Verification items for the finished model (mm, model axes). A direction names the side the tool comes from. Round coordinates to 2 decimals unless told otherwise and drop trailing zeros. Write each loop counter-clockwise with the first axis right and the second up, starting at its lowest first coordinate (ties: lowest second). Pieces come first, ordered by that corner, then holes. Notation, with made-up numbers: M 32,17.25 L 58,17.25 A36 cw 58,52.25 Z; hole C -23,26 d3. An arc over 180 degrees is marked long. One line per question, with ' | ' between items. Start each with the question number.
Q1. Thickness scan on line 1 along Z through (x, y) = (7, -0.3); line 2 along X through (y, z) = (0.5, 9.25); line 3 along X through (y, z) = (11, 3). Record the ranges inside material, lowest first. Write a range as from..to.
Q2. Cross-section at D-D (y = 8). Record the boundary of the cut face in (x, z), then the cut area to 3 significant figures.
Q3. Cross-section at A-A (z = 7.5). State how many separate pieces and enclosed holes the cut face has, then the cut area to 3 significant figures.
Q4. Cross-section at B-B (x = -7.75). Record the boundary of the cut face in (y, z), then the cut area to 3 significant figures.
Q5. Cross-section at C-C (z = 1). Record the boundary of the cut face in (x, y).
Q6. Gauge pin test, flat ends, axial feed: pin 1 (8 mm diameter, centred on x = -7.5, z = 9, fed in from -Y); pin 2 (3.5 mm diameter, centred on y = 9, z = 6, fed in from -X); pin 3 (3 mm diameter, centred on y = 18, z = 2, fed in from -X); pin 4 (3 mm diameter, centred on y = 19.5, z = 7.5, fed in from -X). Record the tip position at first contact, or that the pin passes through.
Q7. Release check for a two-part mould opening along X. For faces 5 (the face through (-0.1, 18.4, 7.4)), 6 (the face through (11, 0, 7)), 7 (the face through (7, 23.5, 7)) record: released by +X, released by -X, zero draft, split by the parting line, or undercut.
Q8. Tool access check on faces 1 (the face through (-3.5, 9, 7)), 2 (the face through (-11, 0, 7)), 3 (the face through (8.18, -0.03, 5.24)), 4 (the face through (9.4, 2, 5.7)). Record the directions out of +Z, -Z, +X, -X, +Y, -Y that give a thin tool (end or side, any length) a straight path to the whole face; none if there is none.
from build123d import *

# Parameters (mm, degrees)
SALIENTE_EXTRUIR1_DEPTH = 15
REDONDEO1_R             = 0.5
REDONDEO2_R             = 0.5
CROQUIS3_R              = 2.55
CORTAR_EXTRUIR1_DEPTH   = 6


with BuildPart() as part:
    # Croquis1 → Saliente-Extruir1 (new body)
    with BuildSketch(Plane.XY):
        with BuildLine():
            Line((-11, 2), (-3.5, 2))
            Line((-3.5, 2), (-3.5, 15.1))
            ThreePointArc((-3.5, 15.1), (-7.571657678, 18.452228214), (-9.1, 23.5))
            Line((-9.1, 23.5), (-5.1, 23.5))
            ThreePointArc((-5.1, 23.5), (0, 18.4), (5.1, 23.5))
            Line((5.1, 23.5), (9.1, 23.5))
            ThreePointArc((9.1, 23.5), (7.571657678, 18.452228214), (3.5, 15.1))
            Line((3.5, 15.1), (3.5, 2))
            Line((3.5, 2), (11, 2))
            Line((11, 2), (11, -2))
            Line((11, -2), (-11, -2))
            Line((-11, -2), (-11, 2))
        make_face()
    extrude(amount=SALIENTE_EXTRUIR1_DEPTH)

    # Redondeo1
    redondeo1_edges = [part.edges().sort_by_distance(p)[0] for p in [
        (-3.5, 2, 7.5),
        (-3.5, 15.1, 7.5),
        (3.5, 15.1, 7.5),
        (3.5, 2, 7.5),
    ]]
    fillet(redondeo1_edges, radius=REDONDEO1_R)

    # Redondeo2
    redondeo2_edges = [part.edges().sort_by_distance(p)[0] for p in [
        (-11, 2, 7.5),
        (-9.1, 23.5, 7.5),
        (-5.1, 23.5, 7.5),
        (5.1, 23.5, 7.5),
        (9.1, 23.5, 7.5),
        (11, 2, 7.5),
    ]]
    fillet(redondeo2_edges, radius=REDONDEO2_R)

    # Croquis3 → Cortar-Extruir1 (cut)
    with BuildSketch(Plane.XZ.offset(2)):
        with Locations(Location((-7, 7.5, 0), (0, 0, 270))):
            Circle(CROQUIS3_R)
        with Locations((7, 7.5)):
            Circle(CROQUIS3_R)
    extrude(amount=-CORTAR_EXTRUIR1_DEPTH, mode=Mode.SUBTRACT)


solid = part.part
Determined:
1) line 1: z = 0..4.95, 10.05..15 | line 2: x = -11..-8.85, -5.15..5.15, 8.85..11 | line 3: x = -3.5..3.5
2) outline: M -3.5,0 L 3.5,0 L 3.5,15 L -3.5,15 Z | area: 105 mm²
3) separate pieces: 3 | enclosed holes: 0 | area: 225 mm²
4) outline: M -2,0 L 2,0 L 2,5.06 L -2,5.06 Z; M -2,9.94 L 2,9.94 L 2,15 L -2,15 Z; M 18.73,0 L 23.5,0 L 23.5,15 L 18.73,15 Z | area: 112 mm²
5) outline: M -11,-2 L 11,-2 L 11,1.5 A0.5 ccw 10.5,2 L 4,2 A0.5 cw 3.5,2.5 L 3.5,14.77 A0.5 cw 3.79,15.23 A9.1 ccw 9.08,22.97 A0.5 ccw 8.59,23.5 L 5.58,23.5 A0.5 ccw 5.08,23.04 A5.1 cw -5.08,23.04 A0.5 ccw -5.58,23.5 L -8.59,23.5 A0.5 ccw -9.08,22.97 A9.1 ccw -3.79,15.23 A0.5 cw -3.5,14.77 L -3.5,2.5 A0.5 cw -4,2 L -10.5,2 A0.5 ccw -11,1.5 Z
6) pin 1: stops at y = -2 | pin 2: stops at x = -3.5 | pin 3: stops at x = -8.17 | pin 4: stops at x = -8.75
7) face 5: undercut | face 6: released by +X | face 7: zero draft
8) face 1: +Z, -Z, -X | face 2: +Z, -Z, -X, +Y, -Y | face 3: -Y | face 4: +Z, -Z, +X
